Design review of the part built by this model. Coordinates are the model's own, in mm. Coordinates: 2 decimals unless noted, no trailing zeros. Loops run counter-clockwise (first coordinate to the right, second up) from the corner with the lowest first, then second, coordinate; pieces in that order, holes last. Notation, with made-up numbers: (67.25, -15) -> (79.25, -15) arc R30 cw to (79.25, 12) -> close; hole circle Ø6 at (-14, -34). An arc over 180 degrees is marked (long way). Answer in a Markdown table with one row per item.
```python
from build123d import *

# Parameters (mm, degrees)
F0_W     = 93.98
F0_H     = 55.88
F1_DEPTH = 0.254
F3_DEPTH = 0.254
F5_DEPTH = 0.254


with BuildPart() as f1:
    # F0 (on Top) → F1 (new body)
    with BuildSketch(Plane.XY):
        with Locations((-3.283079, -18.023962)):
            Rectangle(F0_W, F0_H)
    extrude(amount=F1_DEPTH)

    # F2 (on face) → F3 (join)
    with BuildSketch(Plane.XY.offset(0.254)):
        Polygon((43.706921, 9.916038), (-50.273079, 9.916038), (-50.273079, -45.963962), (43.706921, -45.963962), (43.706921, -44.693962), (-49.003079, -44.693962), (-49.003079, 8.646038), (43.706921, 8.646038), align=None)
    extrude(amount=F3_DEPTH)

    # F4 (on face) → F5 (join)
    with BuildSketch(Plane.XY.offset(0.508)):
        Polygon((-50.273079, 9.916038), (-50.273079, -45.963962), (43.706921, -45.963962), (43.706921, -44.693962), (43.706921, 8.646038), (43.706921, 9.916038), align=None)
    extrude(amount=F5_DEPTH)


solid = f1.part
```
(1) Take a section at A-A on x = 12. Give the boundary of the cut face in (y, z), and give its area (3 significant figures).
Evaluation:
| item | result |
|---|---|
| outline | (-45.96, 0) -> (9.92, 0) -> (9.92, 0.76) -> (-45.96, 0.76) -> close; hole (-44.69, 0.25) -> (8.65, 0.25) -> (8.65, 0.51) -> (-44.69, 0.51) -> close |
| area | 29.0 mm² |
(2) Draft analysis for pull direction Z (two halves, no side actions). For faces 1 (the flat face through (-4, -18, 0.762)), 2 (the flat face through (-4, -18, 0)), 3 (the flat face through (-3, -18, 0.508)), state which applies: pulls with the +Z half, pulls with the -Z half, needs draft (parallel to the pull), parting line crosses it, or undercut.
Evaluation:
| item | result |
|---|---|
| face 1 | pulls with the +Z half |
| face 2 | pulls with the -Z half |
| face 3 | undercut |
(3) Take a section at B-B on y = -13. Give the boundary of the cut face in (x, z).
Evaluation:
| item | result |
|---|---|
| outline | (-50.27, 0) -> (43.71, 0) -> (43.71, 0.25) -> (-49, 0.25) -> (-49, 0.51) -> (43.71, 0.51) -> (43.71, 0.76) -> (-50.27, 0.76) -> close |
(4) To check wall thickness, follow probe 1 along Z at (x, y) = (-45, 7); probe 2 along Y at (x, z) = (-24.5, 0.4); probe 3 along X at (y, z) = (-31, 0.45). State the ranges of each line that lie inside material, in increasing order.
Evaluation:
| item | result |
|---|---|
| probe 1 | z = 0 to 0.25, 0.51 to 0.76 |
| probe 2 | y = -45.96 to -44.69, 8.65 to 9.92 |
| probe 3 | x = -50.27 to -49 |
